Part model, mm, in its own coordinate system. Give positions to 0.01 mm unless a question says otherwise; leave off trailing zeros. Loops run counter-clockwise (first coordinate to the right, second up) from the corner with the lowest first, then second, coordinate; pieces in that order, holes last. Notation, with made-up numbers: (65.25, -25.75) -> (76.25, -25.75) arc R20 ccw to (76.25, 1.25) -> close; hole circle Ø4 at (26.25, 88.5). An arc over 180 degrees is marked (long way). Write item = value, one per line.
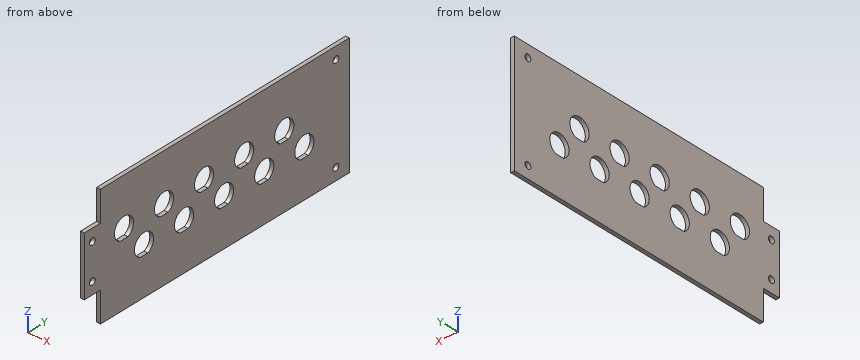
from build123d import *

# Parameters (mm, degrees)
SKETCH1_W           = 14.9
SKETCH1_H           = 49.5
SKETCH1_R           = 2.75
SKETCH1_W_2         = 230
SKETCH1_H_2         = 99.8
BOSS_EXTRUDE1_DEPTH = 3.175
CUT_EXTRUDE1_DEPTH  = 140.190878383


with BuildPart() as part:
    # Sketch1 → Boss-Extrude1 (new body)
    # profile 1 of 2: a face of its own
    with BuildSketch(Plane.YZ):
        with Locations((-122.45, 0)):
            Rectangle(SKETCH1_W, SKETCH1_H)
        with Locations(Location((-122.5, -14.75, 0), (0, 0, 270))):
            Circle(SKETCH1_R, mode=Mode.SUBTRACT)
        with Locations(Location((-122.5, 14.75, 0), (0, 0, 270))):
            Circle(SKETCH1_R, mode=Mode.SUBTRACT)
    # profile 2 of 2: a face of its own
    with BuildSketch(Plane.YZ):
        Rectangle(SKETCH1_W_2, SKETCH1_H_2)
        with Locations(Location((102.5, -39.9, 0), (0, 0, 270))):
            Circle(SKETCH1_R, mode=Mode.SUBTRACT)
        with Locations(Location((102.5, 39.9, 0), (0, 0, 270))):
            Circle(SKETCH1_R, mode=Mode.SUBTRACT)
    extrude(amount=BOSS_EXTRUDE1_DEPTH)

    # Sketch2 → Cut-Extrude1 (cut, through all)
    with BuildSketch(Plane.YZ.offset(3.175)):
        with BuildLine():
            Line((51.1685143, 2.4228), (58.473299942, 2.4228))
            ThreePointArc((58.473299942, 2.4228), (54.820907121, 19.3646), (51.1685143, 2.4228))
        make_face()
        with BuildLine():
            Line((69.688773477, -18.5772), (76.99355912, -18.5772))
            ThreePointArc((76.99355912, -18.5772), (73.341166299, -1.6354), (69.688773477, -18.5772))
        make_face()
        with BuildLine():
            Line((14.127995945, 2.4228), (21.432781587, 2.4228))
            ThreePointArc((21.432781587, 2.4228), (17.780388766, 19.3646), (14.127995945, 2.4228))
        make_face()
        with BuildLine():
            Line((32.648255122, -18.5772), (39.953040765, -18.5772))
            ThreePointArc((39.953040765, -18.5772), (36.300647944, -1.6354), (32.648255122, -18.5772))
        make_face()
        with BuildLine():
            Line((-22.91252241, 2.4228), (-15.607736768, 2.4228))
            ThreePointArc((-15.607736768, 2.4228), (-19.260129589, 19.3646), (-22.91252241, 2.4228))
        make_face()
        with BuildLine():
            Line((-4.392263232, -18.5772), (2.91252241, -18.5772))
            ThreePointArc((2.91252241, -18.5772), (-0.739870411, -1.6354), (-4.392263232, -18.5772))
        make_face()
        with BuildLine():
            Line((-59.953040765, 2.4228), (-52.648255122, 2.4228))
            ThreePointArc((-52.648255122, 2.4228), (-56.300647944, 19.3646), (-59.953040765, 2.4228))
        make_face()
        with BuildLine():
            Line((-41.432781587, -18.5772), (-34.127995945, -18.5772))
            ThreePointArc((-34.127995945, -18.5772), (-37.780388766, -1.6354), (-41.432781587, -18.5772))
        make_face()
        with BuildLine():
            Line((-96.99355912, 2.4228), (-89.688773477, 2.4228))
            ThreePointArc((-89.688773477, 2.4228), (-93.341166299, 19.3646), (-96.99355912, 2.4228))
        make_face()
        with BuildLine():
            Line((-78.473299942, -18.5772), (-71.1685143, -18.5772))
            ThreePointArc((-71.1685143, -18.5772), (-74.820907121, -1.6354), (-78.473299942, -18.5772))
        make_face()
    extrude(amount=-CUT_EXTRUDE1_DEPTH, mode=Mode.SUBTRACT)


solid = part.part
1) Slice it at A-A, the plane z = -39.9. List the corners of the cut face in (x, y) (3 decimals).
Resolved:
outline = (0, -115) -> (3.175, -115) -> (3.175, 99.75) -> (0, 99.75) -> close; (0, 105.25) -> (3.175, 105.25) -> (3.175, 115) -> (0, 115) -> close
2) Drill centre lines: line 1 along Y through (x, z) = (2.5, -10.5); line 2 along Y through (x, z) = (2.4, 10.5); line 3 along Y through (x, z) = (2.45, -37). Where is each one in solid material? Low to high. Write a range as [from, to].
Resolved:
line_1 = [-129.9, -83.69], [-65.96, -46.64], [-28.92, -9.6], [8.12, 27.44], [45.17, 64.48], [82.21, 115]
line_2 = [-129.9, -102.21], [-84.48, -65.17], [-47.44, -28.12], [-10.4, 8.92], [26.64, 45.96], [63.69, 115]
line_3 = [-115, 115]
3) Slice it at B-B, the plane y = 102.5. List the corners of the cut face in (x, z) (3 decimals).
Resolved:
outline = (0, -49.9) -> (3.175, -49.9) -> (3.175, -42.65) -> (0, -42.65) -> close; (0, -37.15) -> (3.175, -37.15) -> (3.175, 37.15) -> (0, 37.15) -> close; (0, 42.65) -> (3.175, 42.65) -> (3.175, 49.9) -> (0, 49.9) -> close
4) Slice it at C-C, the plane x = 1.5. Count the separate pieces of the cut face and the enclosed holes in it, and give its area (3 significant figures).
Resolved:
separate_pieces = 1
enclosed_holes = 14
area = 21,200 mm²
5) Drop a flat-ended pin along its axis: P1, Ø1, axis at x = 1, y = -119, coming from the -Z side. Give the stop position or say it passes through.
Resolved:
P1 = -24.75
